```python
from build123d import *

# Parameters (mm, degrees)
F1_DEPTH = 11.1125


# Not quite as in the source:
# - a length typed as a fraction of an inch, garbled in the dataset ("3 / 203.2 mm" for 3/8 in), is restored


with BuildPart() as f1:
    # F0 (on Top) → F1 (new body)
    with BuildSketch(Plane.XY):
        with BuildLine():
            ThreePointArc((0, 27.0671695471), (-4.5048536548, 25.1556778504), (-8.2258973271, 21.977417171))
            ThreePointArc((-8.2258973271, 21.977417171), (-9.7181261566, 18.698842434), (-9.2097157612, 15.1327075437))
            ThreePointArc((-9.2097157612, 15.1327075437), (-10.6205392688, 11.8246856933), (-10.2093555033, 8.2519613206))
            Line((-10.2093555033, 8.2519613206), (-12.369341217, 7.1464567445))
            Line((-12.369341217, 7.1464567445), (-12.369341217, 4.6386048198))
            Line((-12.369341217, 4.6386048198), (-12.369341217, 4.5682978211))
            ThreePointArc((-12.369341217, 4.5682978211), (-15.5930977879, 3.1185654947), (-17.7027139134, 0.2823972963))
            ThreePointArc((-17.7027139134, 0.2823972963), (-21.0452825194, -1.0603738309), (-23.1384971151, -3.9919692741))
            ThreePointArc((-23.1384971151, -3.9919692741), (-26.5647165348, -5.2934051439), (-28.80180468, -8.19653302))
            ThreePointArc((-28.80180468, -8.19653302), (-29.7673344436, -12.5572908836), (-29.5614041388, -17.0189104974))
            ThreePointArc((-29.5614041388, -17.0189104974), (-25.7783661022, -19.4669407743), (-21.4921734029, -20.8571857766))
            ThreePointArc((-21.4921734029, -20.8571857766), (-17.8594468391, -20.3713745504), (-15.0192606046, -18.054899429))
            ThreePointArc((-15.0192606046, -18.054899429), (-11.4338171794, -17.7079201351), (-8.5996589687, -15.484556372))
            ThreePointArc((-8.5996589687, -15.484556372), (-5.0294162563, -15.0523544446), (-2.1409380715, -12.9098966718))
            Line((-2.1409380715, -12.9098966718), (0, -14.2561570176))
            Line((0, -14.2561570176), (1.9696742658, -12.9098966718))
            ThreePointArc((1.9696742658, -12.9098966718), (4.9392756736, -15.0084468105), (8.560301624, -15.3410370587))
            ThreePointArc((8.560301624, -15.3410370587), (11.3944598347, -17.5644008218), (14.9799032599, -17.9113801157))
            ThreePointArc((14.9799032599, -17.9113801157), (19.5156578324, -16.3470620723), (23.423301056, -13.563092798))
            ThreePointArc((23.423301056, -13.563092798), (23.8861103651, -8.6849198531), (23.0991397704, -3.8484499608))
            ThreePointArc((23.0991397704, -3.8484499608), (21.0059251747, -0.9168545176), (17.6633565687, 0.4259166096))
            ThreePointArc((17.6633565687, 0.4259166096), (15.4847616458, 3.3168082822), (12.1560195839, 4.739132713))
            Line((12.1560195839, 4.739132713), (12.1560195839, 7.1464567445))
            Line((12.1560195839, 7.1464567445), (9.9960338703, 8.2519613206))
            ThreePointArc((9.9960338703, 8.2519613206), (10.4072176357, 11.8246856933), (8.9963941282, 15.1327075437))
            ThreePointArc((8.9963941282, 15.1327075437), (9.5048045235, 18.698842434), (8.012575694, 21.977417171))
            ThreePointArc((8.012575694, 21.977417171), (4.4155385291, 25.1665589), (0, 27.0671695471))
        make_face()
    extrude(amount=F1_DEPTH)


solid = f1.part
```
Can you work these out from the model? Positions are in its coordinate system, mm. A direction names the side the tool comes from. Round coordinates to 2 decimals unless told otherwise and drop trailing zeros. Loops run counter-clockwise (first coordinate to the right, second up) from the corner with the lowest first, then second, coordinate; pieces in that order, holes last.
Item 1: Suppose I cut it at C-C, the plane y = 14. Write out the boundary of the cut face in (x, z), then the cut area to 3 significant figures.
Item 2: Suppose I cut it at B-B, the plane x = -11.5. Write out the boundary of the cut face in (y, z), then the cut area to 3 significant figures.
Item 3: If we mould it in two halves opening along Y, with no side actions, what happens to faces 1 (the cylindrical face through (4.47, 25.13, 5.48)), 2 (the flat face through (-12.369, 6, 5)), 3 (the cylindrical face through (-9.71, 18.75, 5.48))? For each: +Y half, -Y half, draft (parallel to the pull), parting line (faces both ways), or undercut.
Item 4: Suppose I cut it at A-A, the plane z = 4.5. Write out the boundary of the cut face in (x, y).
Item 5: Please list where these lines run through material, in increasing order: L1, parallel to X at y = -13, z = 1.25; L2, parallel to Y at x = 7, z = 6.5; L3, parallel to Y at x = -19, z = 4.25.
Item 6: Will these pins go through, and if not, where does the flat tip stop? pin 1 Ø1.9 at (y, z) = (6, 5) entering from +X; pin 2 Ø1 at (y, z) = (-2.5, 8) entering from +X; pin 3 Ø1.5 at (x, z) = (-3, 4) entering from -Y.
Item 7: Which directions (+Z, -Z, +X, -X, +Y, -Y) give clear straight access to the entire face, cutting with the end or side of a thin tool? Please do faces 4 (the flat face through (-1.09, -13.57, 5.48)), 5 (the flat face through (12.156, 6, 5)), 6 (the flat face through (11.09, 7.69, 5.48)), 7 (the cylindrical face through (-4.45, 25.19, 5.48)).
Reported:
1. outline: (-9.93, 0) - (9.72, 0) - (9.72, 11.11) - (-9.93, 11.11) - close
1. area: 218 mm2
2. outline: (-17.73, 0) - (7.59, 0) - (7.59, 11.11) - (-17.73, 11.11) - close
2. area: 281 mm2
3. face 1: +Y half
3. face 2: draft
3. face 3: undercut
4. outline: (-29.56, -17.02) arc R17.33 ccw to (-21.49, -20.86) arc R6.73 ccw to (-15.02, -18.05) arc R6.42 ccw to (-8.6, -15.48) arc R7.02 ccw to (-2.14, -12.91) - (0, -14.26) - (1.97, -12.91) arc R7.02 ccw to (8.56, -15.34) arc R6.42 ccw to (14.98, -17.91) arc R16.78 ccw to (23.42, -13.56) arc R19.2 ccw to (23.1, -3.85) arc R6.42 ccw to (17.66, 0.43) arc R7.02 ccw to (12.16, 4.74) - (12.16, 7.15) - (10, 8.25) arc R7.02 ccw to (9, 15.13) arc R6.42 ccw to (8.01, 21.98) arc R15.14 ccw to (0, 27.07) arc R16.08 ccw to (-8.23, 21.98) arc R6.42 ccw to (-9.21, 15.13) arc R7.02 ccw to (-10.21, 8.25) - (-12.37, 7.15) - (-12.37, 4.57) arc R7.02 ccw to (-17.7, 0.28) arc R6.42 ccw to (-23.14, -3.99) arc R6.73 ccw to (-28.8, -8.2) arc R16.97 ccw to start
5. L1: x = -29.8 to -2.21, -2 to 1.84, 2.05 to 23.54
5. L2: y = -15.43 to 23.1
5. L3: y = -20.75 to 0.02
6. pin 1: stops at x = 12.16
6. pin 2: stops at x = 22.73
6. pin 3: stops at y = -14.38
7. face 4: +Z, -Z, -Y
7. face 5: +Z, -Z, +X, +Y
7. face 6: +Z, -Z, +X
7. face 7: +Z, -Z, -X, +Y
